```python
from build123d import *

# Parameters (mm, degrees)
F1_DEPTH = 13
F2_DEPTH = 1.6
F3_START = -12
F3_DEPTH = 3
F4_START = -12
F0_W     = 17.8
F0_H     = 7.2
F4_DEPTH = 19


with BuildPart() as f1:
    # F0 (on Right) → F1 (new body)
    with BuildSketch(Plane.YZ):
        with BuildLine():
            Line((37.7, 8.983691223), (-36.7, 8.983691223))
            Line((-36.7, 8.983691223), (-37.7, 8.983691223))
            ThreePointArc((-37.7, 8.983691223), (-39.1142135624, 8.3979047853), (-39.7, 6.983691223))
            Line((-39.7, 6.983691223), (-39.7, 5.983691223))
            Line((-39.7, 5.983691223), (-39.7, -6.983691223))
            ThreePointArc((-39.7, -6.983691223), (-39.1142135624, -8.3979047853), (-37.7, -8.983691223))
            Line((-37.7, -8.983691223), (37.7, -8.983691223))
            ThreePointArc((37.7, -8.983691223), (39.1142135624, -8.3979047853), (39.7, -6.983691223))
            Line((39.7, -6.983691223), (39.7, 6.983691223))
            ThreePointArc((39.7, 6.983691223), (39.1142135624, 8.3979047853), (37.7, 8.983691223))
        make_face()
        with BuildLine():
            Line((37.2, -8.45), (-37.2, -8.45))
            ThreePointArc((-37.2, -8.45), (-38.2606601718, -8.0106601718), (-38.7, -6.95))
            Line((-38.7, -6.95), (-38.7, 6.95))
            ThreePointArc((-38.7, 6.95), (-38.2606601718, 8.0106601718), (-37.2, 8.45))
            Line((-37.2, 8.45), (37.2, 8.45))
            ThreePointArc((37.2, 8.45), (38.2606601718, 8.0106601718), (38.7, 6.95))
            Line((38.7, 6.95), (38.7, -6.95))
            ThreePointArc((38.7, -6.95), (38.2606601718, -8.0106601718), (37.2, -8.45))
        make_face(mode=Mode.SUBTRACT)
    extrude(amount=-F1_DEPTH)

    # F0 (on Right) → F2 (join)
    with BuildSketch(Plane.YZ):
        with BuildLine():
            ThreePointArc((-41.17091404, -6.71898761), (-39.9993411647, -9.5474147347), (-37.17091404, -10.71898761))
            Line((-37.17091404, -10.71898761), (37.99908596, -10.71898761))
            ThreePointArc((37.99908596, -10.71898761), (40.8275130848, -9.5474147347), (41.99908596, -6.71898761))
            Line((41.99908596, -6.71898761), (41.99908596, 5.884703613))
            ThreePointArc((41.99908596, 5.884703613), (40.8275130848, 8.7131307377), (37.99908596, 9.884703613))
            Line((37.99908596, 9.884703613), (-37.17091404, 9.884703613))
            ThreePointArc((-37.17091404, 9.884703613), (-39.9993411647, 8.7131307377), (-41.17091404, 5.884703613))
            Line((-41.17091404, 5.884703613), (-41.17091404, -6.71898761))
        make_face()
        with BuildLine():
            Line((-37.7, 8.983691223), (-36.7, 8.983691223))
            Line((-36.7, 8.983691223), (37.7, 8.983691223))
            ThreePointArc((37.7, 8.983691223), (39.1142135624, 8.3979047853), (39.7, 6.983691223))
            Line((39.7, 6.983691223), (39.7, -6.983691223))
            ThreePointArc((39.7, -6.983691223), (39.1142135624, -8.3979047853), (37.7, -8.983691223))
            Line((37.7, -8.983691223), (-37.7, -8.983691223))
            ThreePointArc((-37.7, -8.983691223), (-39.1142135624, -8.3979047853), (-39.7, -6.983691223))
            Line((-39.7, -6.983691223), (-39.7, 5.983691223))
            Line((-39.7, 5.983691223), (-39.7, 6.983691223))
            ThreePointArc((-39.7, 6.983691223), (-39.1142135624, 8.3979047853), (-37.7, 8.983691223))
        make_face(mode=Mode.SUBTRACT)
        with BuildLine():
            Line((37.7, 8.983691223), (-36.7, 8.983691223))
            Line((-36.7, 8.983691223), (-37.7, 8.983691223))
            ThreePointArc((-37.7, 8.983691223), (-39.1142135624, 8.3979047853), (-39.7, 6.983691223))
            Line((-39.7, 6.983691223), (-39.7, 5.983691223))
            Line((-39.7, 5.983691223), (-39.7, -6.983691223))
            ThreePointArc((-39.7, -6.983691223), (-39.1142135624, -8.3979047853), (-37.7, -8.983691223))
            Line((-37.7, -8.983691223), (37.7, -8.983691223))
            ThreePointArc((37.7, -8.983691223), (39.1142135624, -8.3979047853), (39.7, -6.983691223))
            Line((39.7, -6.983691223), (39.7, 6.983691223))
            ThreePointArc((39.7, 6.983691223), (39.1142135624, 8.3979047853), (37.7, 8.983691223))
        make_face()
        with BuildLine():
            Line((37.2, -8.45), (-37.2, -8.45))
            ThreePointArc((-37.2, -8.45), (-38.2606601718, -8.0106601718), (-38.7, -6.95))
            Line((-38.7, -6.95), (-38.7, 6.95))
            ThreePointArc((-38.7, 6.95), (-38.2606601718, 8.0106601718), (-37.2, 8.45))
            Line((-37.2, 8.45), (37.2, 8.45))
            ThreePointArc((37.2, 8.45), (38.2606601718, 8.0106601718), (38.7, 6.95))
            Line((38.7, 6.95), (38.7, -6.95))
            ThreePointArc((38.7, -6.95), (38.2606601718, -8.0106601718), (37.2, -8.45))
        make_face(mode=Mode.SUBTRACT)
    extrude(amount=F2_DEPTH)

    # F0 (on Right) → F3 (join)
    with BuildSketch(Plane.YZ.offset(F3_START)):
        with BuildLine():
            Line((37.7, 8.983691223), (-36.7, 8.983691223))
            Line((-36.7, 8.983691223), (-37.7, 8.983691223))
            ThreePointArc((-37.7, 8.983691223), (-39.1142135624, 8.3979047853), (-39.7, 6.983691223))
            Line((-39.7, 6.983691223), (-39.7, 5.983691223))
            Line((-39.7, 5.983691223), (-39.7, -6.983691223))
            ThreePointArc((-39.7, -6.983691223), (-39.1142135624, -8.3979047853), (-37.7, -8.983691223))
            Line((-37.7, -8.983691223), (37.7, -8.983691223))
            ThreePointArc((37.7, -8.983691223), (39.1142135624, -8.3979047853), (39.7, -6.983691223))
            Line((39.7, -6.983691223), (39.7, 6.983691223))
            ThreePointArc((39.7, 6.983691223), (39.1142135624, 8.3979047853), (37.7, 8.983691223))
        make_face()
        with BuildLine():
            Line((37.2, -8.45), (-37.2, -8.45))
            ThreePointArc((-37.2, -8.45), (-38.2606601718, -8.0106601718), (-38.7, -6.95))
            Line((-38.7, -6.95), (-38.7, 6.95))
            ThreePointArc((-38.7, 6.95), (-38.2606601718, 8.0106601718), (-37.2, 8.45))
            Line((-37.2, 8.45), (37.2, 8.45))
            ThreePointArc((37.2, 8.45), (38.2606601718, 8.0106601718), (38.7, 6.95))
            Line((38.7, 6.95), (38.7, -6.95))
            ThreePointArc((38.7, -6.95), (38.2606601718, -8.0106601718), (37.2, -8.45))
        make_face(mode=Mode.SUBTRACT)
        with BuildLine():
            ThreePointArc((-38.7, -6.95), (-38.2606601718, -8.0106601718), (-37.2, -8.45))
            Line((-37.2, -8.45), (37.2, -8.45))
            ThreePointArc((37.2, -8.45), (38.2606601718, -8.0106601718), (38.7, -6.95))
            Line((38.7, -6.95), (38.7, 6.95))
            ThreePointArc((38.7, 6.95), (38.2606601718, 8.0106601718), (37.2, 8.45))
            Line((37.2, 8.45), (-37.2, 8.45))
            ThreePointArc((-37.2, 8.45), (-38.2606601718, 8.0106601718), (-38.7, 6.95))
            Line((-38.7, 6.95), (-38.7, -6.95))
        make_face()
        with BuildLine():
            ThreePointArc((10.8, -1.3001189455), (10.2142135624, -2.7143325079), (8.8, -3.3001189455))
            Line((8.8, -3.3001189455), (-8.8, -3.3001189455))
            ThreePointArc((-8.8, -3.3001189455), (-10.2142135624, -2.7143325079), (-10.8, -1.3001189455))
            Line((-10.8, -1.3001189455), (-10.8, 4.6998810545))
            ThreePointArc((-10.8, 4.6998810545), (-10.2142135624, 6.1140946168), (-8.8, 6.6998810545))
            Line((-8.8, 6.6998810545), (8.8, 6.6998810545))
            ThreePointArc((8.8, 6.6998810545), (10.2142135624, 6.1140946168), (10.8, 4.6998810545))
            Line((10.8, 4.6998810545), (10.8, -1.3001189455))
        make_face(mode=Mode.SUBTRACT)
    extrude(amount=-F3_DEPTH)

    # F0 (on Right) → F4 (join)
    with BuildSketch(Plane.YZ.offset(F4_START)):
        with BuildLine():
            Line((-8.8, -3.3001189455), (8.8, -3.3001189455))
            ThreePointArc((8.8, -3.3001189455), (10.2142135624, -2.7143325079), (10.8, -1.3001189455))
            Line((10.8, -1.3001189455), (10.8, 4.6998810545))
            ThreePointArc((10.8, 4.6998810545), (10.2142135624, 6.1140946168), (8.8, 6.6998810545))
            Line((8.8, 6.6998810545), (-8.8, 6.6998810545))
            ThreePointArc((-8.8, 6.6998810545), (-10.2142135624, 6.1140946168), (-10.8, 4.6998810545))
            Line((-10.8, 4.6998810545), (-10.8, -1.3001189455))
            ThreePointArc((-10.8, -1.3001189455), (-10.2142135624, -2.7143325079), (-8.8, -3.3001189455))
        make_face()
        with Locations((0, 1.6998810545)):
            Rectangle(F0_W, F0_H, mode=Mode.SUBTRACT)
    extrude(amount=-F4_DEPTH)


solid = f1.part
```
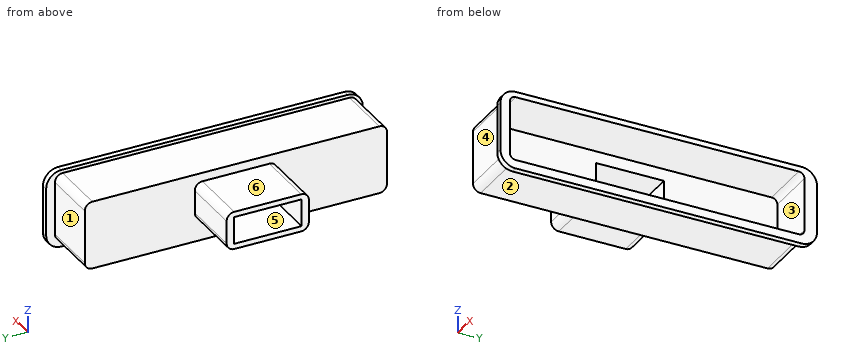
Work out the finished part from the listing and answer in its coordinate system (mm). Face numbers are marked on the shaded views. A direction names the side the tool comes from. Coordinates: 2 decimals unless noted, no trailing zeros. Write each loop counter-clockwise with the first axis right and the second up, starting at its lowest first coordinate (ties: lowest second). Pieces come first, ordered by that corner, then holes.
Q1. A cutting plane is placed at B-B, the plane y = 7.5. Give the vertices of the cut face in (x, z), then the cut area to 3 significant figures.
Q2. Each of these flat-tipped pins is pushed along its axis until it touches: pin 1 Ø1.5 at (x, y) = (-2, -17) entering from -Z; pin 2 Ø3 at (x, z) = (-22.5, -4.5) entering from -Y; pin 3 Ø6 at (y, z) = (6.5, 4.5) entering from -X; pin 4 Ø12 at (x, y) = (-22, -16.5) entering from -Z. Where does it stop, or does it pass through?
Q3. Which of the six approach directions +Z, -Z, +X, -X, +Y, -Y give full straight-line access (tool end or side, diameter ignored) to the marked faces 1, 2 and 3?
Q4. A cutting plane is placed at D-D, the plane z = -5.5. Give the vertices of the cut face in (x, y).
Q5. Find the intervals of material crossed by line 1 (Y direction, x = -16, z = 3.5); line 2 (Y direction, x = -14.5, z = 5); line 3 (Z direction, x = -0.5, y = 21), in increasing order.
Q6. Determine the mould class of the marked faces 4, 5 and 6 for opening direction Y: released by +Y, released by -Y, zero draft, split by the parting line, or undercut.
Q7. A cutting plane is placed at C-C, the plane x = -24.5. Give the vertices of the cut face in (y, z).
Q8. A cutting plane is placed at A-A, the plane z = 1.25. Give the vertices of the cut face in (x, y).
Findings below:
1. outline: (-31, -3.3) - (-15, -3.3) - (-15, -8.98) - (0, -8.98) - (0, -10.72) - (1.6, -10.72) - (1.6, -8.45) - (-12, -8.45) - (-12, -1.9) - (-31, -1.9) - close; (-31, 5.3) - (-12, 5.3) - (-12, 8.45) - (1.6, 8.45) - (1.6, 9.88) - (0, 9.88) - (0, 8.98) - (-15, 8.98) - (-15, 6.7) - (-31, 6.7) - close
1. area: 95.8 mm2
2. pin 1: stops at z = -8.98
2. pin 2: stops at y = -9.85
2. pin 3: stops at x = -31
2. pin 4: stops at z = -2.35
3. face 1: +Z, -Z, -X, +Y
3. face 2: -Z, -X, +Y, -Y
3. face 3: +X
4. outline: (-15, -39.7) - (0, -39.7) - (0, -41.17) - (1.6, -41.17) - (1.6, -38.7) - (-12, -38.7) - (-12, 38.7) - (1.6, 38.7) - (1.6, 42) - (0, 42) - (0, 39.7) - (-15, 39.7) - close
5. line 1: y = -10.8 to -8.9, 8.9 to 10.8
5. line 2: y = -39.7 to -8.9, 8.9 to 39.7
5. line 3: z = -8.98 to -8.45, 8.45 to 8.98
6. face 4: released by -Y
6. face 5: undercut
6. face 6: zero draft
7. outline: (-10.8, -1.3) arc R2 ccw to (-8.8, -3.3) - (8.8, -3.3) arc R2 ccw to (10.8, -1.3) - (10.8, 4.7) arc R2 ccw to (8.8, 6.7) - (-8.8, 6.7) arc R2 ccw to (-10.8, 4.7) - close; hole (-8.9, -1.9) - (8.9, -1.9) - (8.9, 5.3) - (-8.9, 5.3) - close
8. outline: (-31, -10.8) - (-15, -10.8) - (-15, -39.7) - (0, -39.7) - (0, -41.17) - (1.6, -41.17) - (1.6, -38.7) - (-12, -38.7) - (-12, -8.9) - (-31, -8.9) - close; (-31, 8.9) - (-12, 8.9) - (-12, 38.7) - (1.6, 38.7) - (1.6, 42) - (0, 42) - (0, 39.7) - (-15, 39.7) - (-15, 10.8) - (-31, 10.8) - close
